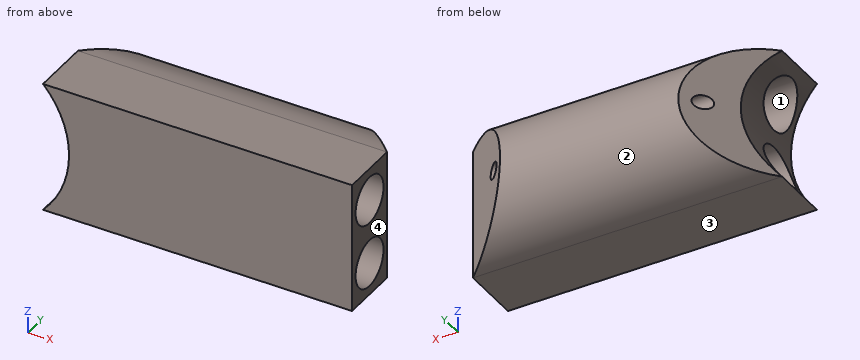
from build123d import *

# Parameters (mm, degrees)
SKETCH1_W              = 33.02
SKETCH1_H              = 13.97
DEPTH_A_DEPTH          = 6.35
ROUND_EXTRUDE_DEPTH    = 33.02
ANGLE_CUT_DEPTH        = 39.253150524
STRING_HOLE_R          = 0.762
STRING_HOLE_CUT_DEPTH  = 39.253150524
ELASTIC_HOLES_R        = 2.54
ELASTIC_HOLE_CUT_DEPTH = 39.253150524
GUIDE_CUT_REACH        = 40.253


with BuildPart() as part:
    # Sketch1 → depth a (new body)
    with BuildSketch(Plane(origin=(0, 0, 0), x_dir=(1, 0, 0), z_dir=(0, 1, 0))):
        with Locations((-16.51, 6.985)):
            Rectangle(SKETCH1_W, SKETCH1_H)
    extrude(amount=DEPTH_A_DEPTH)

    # Sketch4 → round extrude (add)
    with BuildSketch(Plane(origin=(0, 0, 0), x_dir=(0, 0, -1), z_dir=(1, 0, 0))):
        with BuildLine():
            Line((0, 6.35), (13.97, 6.35))
            ThreePointArc((13.97, 6.35), (6.985, 13.335), (0, 6.35))
        make_face()
    extrude(amount=-ROUND_EXTRUDE_DEPTH)

    # Sketch5 → angle cut (cut, through all)
    with BuildSketch(Plane.XY):
        Polygon((0, 6.35), (0, 13.335), (-6.985, 13.335), align=None)
        Polygon((-33.02, 6.35), (-33.02, 13.335), (-26.035, 13.335), align=None)
    extrude(amount=-ANGLE_CUT_DEPTH, mode=Mode.SUBTRACT)

    # string hole → string hole cut (cut, through all)
    with BuildSketch(Plane(origin=(0, 0, 0), x_dir=(0, 0, -1), z_dir=(1, 0, 0))):
        with Locations(Location((6.985, 11.684, 0), (0, 0, 270))):
            Circle(STRING_HOLE_R)
    extrude(amount=-STRING_HOLE_CUT_DEPTH, mode=Mode.SUBTRACT)

    # elastic holes → elastic hole cut (cut, through all)
    with BuildSketch(Plane(origin=(0, 0, 0), x_dir=(0, 0, -1), z_dir=(1, 0, 0))):
        with Locations((3.4925, 3.175)):
            Circle(ELASTIC_HOLES_R)
        with Locations(Location((10.4775, 3.175, 0), (0, 0, 180))):
            Circle(ELASTIC_HOLES_R)
    extrude(amount=-ELASTIC_HOLE_CUT_DEPTH, mode=Mode.SUBTRACT)

    # guide → guide cut (cut, up to next)
    with BuildSketch(Plane(origin=(0, 0, 0), x_dir=(1, 0, 0), z_dir=(0, 1, 0)), mode=Mode.PRIVATE) as guide_cut_sk1:
        with BuildLine():
            Line((-33.02, 13.97), (-33.02, 0))
            ThreePointArc((-33.02, 0), (-30.238033275, 6.985), (-33.02, 13.97))
        make_face()
    guide_cut_tool1 = extrude(guide_cut_sk1.sketch, amount=GUIDE_CUT_REACH, mode=Mode.PRIVATE) & part.part
    add(guide_cut_tool1.solids().sort_by_distance((-31.893025, 0, -6.985))[0], mode=Mode.SUBTRACT)


solid = part.part
For this review, take the finished solid that the model builds, in its own axes (mm). Face numbers are marked on the shaded views. Round coordinates to 2 decimals unless told otherwise and drop trailing zeros. Loops run counter-clockwise (first coordinate to the right, second up) from the corner with the lowest first, then second, coordinate; pieces in that order, holes last. Notation, with made-up numbers: (55.5, 4) - (79.5, 4) arc R29 ccw to (79.5, 41) - close; hole circle Ø9 at (43.5, -37). An arc over 180 degrees is marked (long way). One line per item, written item: value. Start each with the question number.
Item 1: Take a section at A-A (z = -8.5). Give the boundary of the cut face in (x, y).
Item 2: Take a section at D-D (y = 2.5). Give the boundary of the cut face in (x, z) (3 decimals), plus the area to 3 significant figures.
Item 3: Clearance check with flat-ended pins moving along their axes: pin 1 Ø2.5 at (y, z) = (11.684, -6.985) entering from +X; pin 2 Ø4 at (x, y) = (-19.5, 11.5) entering from +Z; pin 3 Ø6 at (y, z) = (7.5, -5) entering from -X. State where each tip first meets the part, or that it passes through.
Item 4: For L1, parallel to Z at x = -2.5, y = 3.25; L2, parallel to Z at x = -13, y = 2; L3, parallel to Y at x = -6.5, z = -2, list the stretches that pass through material, from the lowest coordinate up.
Item 5: The part is to be moulded in two halves that separate along Z. For the marked faces 1, 2, 3 and 4, say which applies: +Z half, -Z half, draft (parallel to the pull), parting line (faces both ways), or undercut.
Item 6: Take a section at B-B (y = 4). Give the boundary of the cut face in (x, z) (3 decimals).
Item 7: Take a section at C-C (x = -21). State how many separate pieces and enclosed holes the cut face has, plus the area to 3 significant figures.
Answer below:
1. outline: (-30.35, 0) - (0, 0) - (0, 1.58) - (-30.35, 1.58) - close; (-30.35, 4.77) - (0, 4.77) - (0, 6.35) - (-6.82, 13.17) - (-26.2, 13.17) - (-30.35, 9.02) - close
2. outline: (-33.02, -13.97) - (0, -13.97) - (0, -12.926) - (-32.156, -12.926) arc R10.16 cw to start; (-33.02, 0) arc R10.16 cw to (-32.156, -1.044) - (0, -1.044) - (0, 0) - close; (-30.292, -8.029) - (0, -8.029) - (0, -5.941) - (-30.292, -5.941) arc R10.16 cw to start
2. area: 131 mm2
3. pin 1: stops at x = -4.08
3. pin 2: stops at z = -0.75
3. pin 3: stops at x = -31.55
4. L1: z = -13.97 to -13.02, -7.94 to -6.03, -0.95 to 0
4. L2: z = -13.97 to -12.73, -8.23 to -5.74, -1.24 to 0
4. L3: y = 0 to 1.12, 5.23 to 11.24
5. face 1: undercut
5. face 2: parting line
5. face 3: -Z half
5. face 4: draft
6. outline: (-33.02, -13.97) - (0, -13.97) - (0, -12.88) - (-32.123, -12.88) arc R10.16 cw to start; (-33.02, 0) arc R10.16 cw to (-32.123, -1.09) - (0, -1.09) - (0, 0) - close; (-30.297, -8.075) - (0, -8.075) - (0, -5.895) - (-30.297, -5.895) arc R10.16 cw to start
7. separate pieces: 1
7. enclosed holes: 3
7. area: 123 mm2
